Read the model definition and answer for the solid it produces. Units are mm, in the model's axes. A direction names the side the tool comes from. Give positions to 0.01 mm unless a question says otherwise; leave off trailing zeros. Order: outer loops, then holes, each group sorted by start corner. A loop starts at its lowest first (then second) coordinate and runs counter-clockwise, first axis right, second up. Notation, with made-up numbers: (-4.75, 63.5) - (2.25, 63.5) arc R31 ccw to (2.25, 90.5) - close; hole circle Ø6 at (-35, -30). An arc over 180 degrees is marked (long way). Write item = value, one per line.
```python
from build123d import *

# Parameters (mm, degrees)
SKETCH1_W           = 120
SKETCH1_H           = 40
SKETCH1_W_2         = 19.98
SKETCH1_H_2         = 9
BOSS_EXTRUDE1_DEPTH = 4.7625
FILLET1_R           = 1


with BuildPart() as part:
    # Sketch1 → Boss-Extrude1 (new, symmetric)
    with BuildSketch(Plane.XY):
        Rectangle(SKETCH1_W, SKETCH1_H)
        with Locations((-24.99, -24.5)):
            Rectangle(SKETCH1_W_2, SKETCH1_H_2)
        with Locations((24.99, -24.5)):
            Rectangle(SKETCH1_W_2, SKETCH1_H_2)
    extrude(amount=BOSS_EXTRUDE1_DEPTH, both=True)

    # Fillet1
    fillet1_edges = [part.edges().sort_by_distance(p)[0] for p in [
        (-60, 20, 0),
        (60, 20, 0),
    ]]
    fillet(fillet1_edges, radius=FILLET1_R)


solid = part.part
```
1. For faces 4 (the face through (47, -20, 0)), 5 (the face through (-15, -25, 0)), 6 (the face through (-34.98, -25, 0)), determine the directions among +Z, -Z, +X, -X, +Y, -Y from which every point of the face is accessible in a straight line to the end or side of a thin tool.
Recorded:
face_4 = +Z, -Z, +X, -Y
face_5 = +Z, -Z, -Y
face_6 = +Z, -Z, -X, -Y
2. Section A-A (y = -23) is taken. Determine the outline of the cut face in (x, z).
Recorded:
outline = (-34.98, -4.76) - (-15, -4.76) - (-15, 4.76) - (-34.98, 4.76) - close; (15, -4.76) - (34.98, -4.76) - (34.98, 4.76) - (15, 4.76) - close
3. Determine the mould class of faces 1 (the face through (34.98, -25, 0)), 2 (the face through (-1, 1, 4.762)), 3 (the face through (15, -25, 0)) for opening direction X: +X half, -X half, draft (parallel to the pull), parting line (faces both ways), or undercut.
Recorded:
face_1 = +X half
face_2 = draft
face_3 = undercut
4. Flat-ended cylindrical pins translate along their axes: pin 1 (2.5 mm diameter, centred on y = -24, z = 2.5, fed in from +X); pin 2 (3 mm diameter, centred on x = 7, z = 1.5, fed in from -Y); pin 3 (1.5 mm diameter, centred on x = -47.5, y = -21, fed in from +Z); pin 4 (1.5 mm diameter, centred on y = -22.5, z = 2.5, fed in from -X). Find the tip coordinate at first contact, or state that the pin passes through.
Recorded:
pin_1 = 34.98
pin_2 = -20
pin_3 = through
pin_4 = -34.98
5. Section C-C (x = 48.5) is taken. Determine the outline of the cut face in (y, z).
Recorded:
outline = (-20, -4.76) - (20, -4.76) - (20, 4.76) - (-20, 4.76) - close
6. A straight line is drawn through the part: L1, parallel to Y at x = 7, z = -4.5. Find the intervals that lie inside material, in ascending order. Write a range as [from, to].
Recorded:
L1 = [-20, 20]
7. Section B-B (z = -1.75) is taken. Determine the outline of the cut face in (x, y), and give its area (3 significant figures).
Recorded:
outline = (-60, -20) - (-34.98, -20) - (-34.98, -29) - (-15, -29) - (-15, -20) - (15, -20) - (15, -29) - (34.98, -29) - (34.98, -20) - (60, -20) - (60, 19) arc R1 ccw to (59, 20) - (-59, 20) arc R1 ccw to (-60, 19) - close
area = 5,160 mm^2
